Build history of the part. All positions in model axes, mm. Round coordinates to 2 decimals unless told otherwise and drop trailing zeros. Order: outer loops, then holes, each group sorted by start corner. A loop starts at its lowest first (then second) coordinate and runs counter-clockwise, first axis right, second up. Notation, with made-up numbers: M 66.25,76 L 105.25,76 A11 cw 105.25,94 Z; hole C -29,36 d2. An arc over 180 degrees is marked long. One line per question, with ' | ' between items. Start each with the question number.
Autodesk Inventor part; units mm, degrees
ref_plane "YZ Plane" through (0, 0, 0) normal (1, 0, 0) x (0, 1, 0)
ref_plane "XZ Plane" through (0, 0, 0) normal (0, 1, 0) x (-1, 0, 0)
ref_plane "XY Plane" through (0, 0, 0) normal (0, 0, 1) x (1, 0, 0)
sketch "Sketch1" plane through (0, 0, 0) normal (0, 0, 1) x (1, 0, 0)
  line L0 (0, 0) -> (0, 22.86)
  line L1 (-304.8, 0) -> (-304.8, 22.86)
  line L2 (-304.8, 22.86) -> (-152.4, 0)
  line L3 (-152.4, 0) -> (0, 22.86)
  line L4 (-304.8, 19.6495) -> (-173.8035, 0)
  line L5 (-130.9965, 0) -> (0, 19.6495)
  line L6 (-173.8035, 0) -> (-152.4, -3.2105)
  line L7 (-130.9965, 0) -> (-152.4, -3.2105)
  line L8 (-304.8, 0) -> (-173.8035, 0)
  line L9 (-130.9965, 0) -> (0, 0)
  line L10 (-152.4, -3.2105) -> (-165.1, -3.2105)
  line L11 (-165.1, -3.2105) -> (-165.1, -1.3055)
  dimension "d0" = 22.86
  dimension "d2" = 304.8
  dimension "d4" = 3.175
  dimension "d5" = 3.175
  dimension "d8" = 12.7
extrude "Extrusion1" add sketch "Sketch1" along normal blind 25.4 contours L5 L7 L6 L4 L1 L2 L3 L0
sketch "Sketch2" plane through (0, 0, 25.4) normal (0, 0, 1) x (1, 0, 0)
  line L0 (0, 19.6495) -> (0, 22.86)
  line L1 (0, 22.86) -> (-152.4, 0)
  line L2 (-152.4, 0) -> (-304.8, 22.86)
  line L3 (-304.8, 22.86) -> (-304.8, 19.6495)
  line L4 (-304.8, 22.86) -> (-304.8, 21.5646)
  line L5 (-304.8, 21.5646) -> (-296.164, 21.5646)
  line L6 (0, 22.86) -> (0, 21.5646)
  line L7 (0, 21.5646) -> (-10.7017, 21.2547)
  point P0 (0, 0)
  dimension "d9" = 1.2954
  dimension "d10" = 1.2954
extrude "Extrusion2" cut sketch "Sketch2" against normal blind 50.8
properties part number "plough"
Item 1: Cut at B-B on z = 9. Write the cut outline in (x, y), then the cut area to 3 significant figures.
Item 2: Cut at A-A on y = 4.25. Write the cut outline in (x, z).
Item 3: Cut at C-C on y = 15.75. Write the cut outline in (x, z), then the cut area to 3 significant figures.
Item 4: Cut at D-D on x = -182. Write the cut outline in (y, z), then the cut area to 3 significant figures.
Item 5: Two-plate mould, pull along X, no slides. Class faces 1 (the face through (-82.54, 10.48, 12.52)), 2 (the face through (-225.288, 10.933, 12.522)), 3 (the face through (-301, 21.565, 13)): +X half, -X half, draft (parallel to the pull), parting line (faces both ways), or undercut.
Item 6: Wall check: line 1 along Y through (x, z) = (-138.5, 12.25) (3 decimals); line 2 along Y through (x, z) = (-33, 14.75). Give the ranges that are in metal, low to high. Write a range as [from, to].
Results found:
1) outline: M -304.8,19.65 L -173.8,0 L -152.4,-3.21 L -131,0 L 0,19.65 L 0,21.56 L -10.7,21.25 L -152.4,0 L -296.16,21.56 L -304.8,21.56 Z | area: 966 mm^2
2) outline: M -202.14,0 L -180.73,0 L -180.73,25.4 L -202.14,25.4 Z; M -124.07,0 L -102.66,0 L -102.66,25.4 L -124.07,25.4 Z
3) outline: M -278.8,0 L -257.4,0 L -257.4,25.4 L -278.8,25.4 Z; M -47.4,0 L -26,0 L -26,25.4 L -47.4,25.4 Z | area: 1,090 mm^2
4) outline: M 1.23,0 L 4.44,0 L 4.44,25.4 L 1.23,25.4 Z | area: 81.5 mm^2
5) face 1: undercut | face 2: undercut | face 3: draft
6) line 1: y = [-1.126, 2.085] | line 2: y = [14.7, 17.91]
